Geometry check sheet. Reference: the model listing, model coordinates, mm. A direction names the side the tool comes from. Round coordinates to 2 decimals unless told otherwise and drop trailing zeros. Order: outer loops, then holes, each group sorted by start corner. A loop starts at its lowest first (then second) coordinate and runs counter-clockwise, first axis right, second up. Notation, with made-up numbers: (32, 89) - (39, 89) arc R16 cw to (39, 119) - close; hole circle Ø4 at (45.25, 13.25). An arc over 180 degrees is marked (long way). Use a Markdown table: item, result. Add a question column.
(1) Section check A-A on y = 20. Give the number of separate pieces and of enclosed holes in the cut face, then the cut area to 3 significant figures.
(2) Gauge pin test, flat ends, axial feed: P1, Ø6, axis at y = 24.5, z = -17.5, coming from the +X side; P2, Ø1.5, axis at y = 22.5, z = -22, coming from the -X side; P3, Ø4, axis at y = 29, z = -3.5, coming from the +X side. Record the tip position at first contact, or that the pin passes through.
(3) Section check B-B on y = 3. Record the boundary of the cut face in (x, z), then the cut area to 3 significant figures.
(4) Mould release check, pull along Y, two halves, no side actions. Record for faces 6 (the face through (5.27, 8.1, -11.44)), 7 (the face through (58, 35, -13)), 8 (the face through (46, 3, -24.75)): released by +Y, released by -Y, zero draft, split by the parting line, or undercut.
(5) Thickness scan on line 1 along Z through (x, y) = (18.5, 3); line 2 along X through (y, z) = (9, -12.25); line 3 along X through (y, z) = (10.5, -19.75). Record the ranges inside material, lowest first. Write a range as [from, to].
(6) Access from +Z, -Z, +X, -X, +Y, -Y to the whole of each face (thin tool, end or side, straight path). Record for faces 1 (the face through (1.25, 2, -13)), 2 (the face through (53.27, 8.1, -11.44)), 3 (the face through (13.5, 13, -4)), 4 (the face through (54.5, 27.3, -15.3)), 5 (the face through (61.5, 13, -4)).
(7) Section check C-C on x = 9.5. Record the boundary of the cut face in (y, z).
```python
from build123d import *

# Parameters (mm, degrees)
SKETCH1_W            = 20
SKETCH1_H            = 26
SKETCH1_W_2          = 1.25
SKETCH1_H_2          = 15
BOSS_EXTRUDE5_DEPTH  = 5
SKETCH3_W            = 7
SKETCH3_H            = 26
BOSS_EXTRUDE6_DEPTH  = 40
CUT_EXTRUDE1_REACH   = 55.696
SKETCH5_R            = 11.2
SKETCH6_W            = 26
SKETCH6_H            = 5
BOSS_EXTRUDE8_DEPTH  = 14
SKETCH8_R            = 12
SKETCH8_R_2          = 7.5
BOSS_EXTRUDE9_DEPTH  = 2.5
SKETCH9_R            = 12
SKETCH9_R_2          = 7.5
BOSS_EXTRUDE10_DEPTH = 2.5
SKETCH7_W            = 12
SKETCH7_H            = 1.25
CUT_EXTRUDE2_DEPTH   = 10


with BuildPart() as part:
    # Sketch1 → Boss-Extrude5 (new body)
    with BuildSketch(Plane(origin=(0, 0, 0), x_dir=(1, 0, 0), z_dir=(0, 1, 0))):
        with Locations((10, 13)):
            Rectangle(SKETCH1_W, SKETCH1_H)
        with Locations((1.875, 13)):
            Rectangle(SKETCH1_W_2, SKETCH1_H_2, mode=Mode.SUBTRACT)
    boss_extrude5 = extrude(amount=BOSS_EXTRUDE5_DEPTH)

    # Sketch3 → Boss-Extrude6 (add)
    with BuildSketch(Plane(origin=(0, 5, 0), x_dir=(1, 0, 0), z_dir=(0, 1, 0))):
        with Locations((10, 13)):
            Rectangle(SKETCH3_W, SKETCH3_H)
    boss_extrude6 = extrude(amount=BOSS_EXTRUDE6_DEPTH)

    # Sketch5 → Cut-Extrude1 (cut, up to next)
    with BuildSketch(Plane(origin=(13.5, 0, 0), x_dir=(0, 0, -1), z_dir=(1, 0, 0)), mode=Mode.PRIVATE) as cut_extrude1_sk1:
        with Locations((13, 20)):
            Circle(SKETCH5_R)
    cut_extrude1_tool1 = extrude(cut_extrude1_sk1.sketch, amount=-CUT_EXTRUDE1_REACH, mode=Mode.PRIVATE) & part.part
    # Sketch5 → Cut-Extrude1 (cut, up to next)
    with BuildSketch(Plane(origin=(13.5, 0, 0), x_dir=(0, 0, -1), z_dir=(1, 0, 0)), mode=Mode.PRIVATE) as cut_extrude1_sk2:
        with BuildLine():
            Line((0, 27.483314774), (0, 45))
            Line((0, 45), (26, 45))
            Line((26, 45), (26, 27.483314774))
            ThreePointArc((26, 27.483314774), (13, 35), (0, 27.483314774))
        make_face()
    cut_extrude1_tool2 = extrude(cut_extrude1_sk2.sketch, amount=-CUT_EXTRUDE1_REACH, mode=Mode.PRIVATE) & part.part
    cut_extrude1_1 = cut_extrude1_tool1.solids().sort_by_distance((13.5, 20, -13))[0]
    add(cut_extrude1_1, mode=Mode.SUBTRACT)
    cut_extrude1_2 = cut_extrude1_tool2.solids().sort_by_distance((13.5, 38.725293, -13))[0]
    add(cut_extrude1_2, mode=Mode.SUBTRACT)
    cut_extrude1 = cut_extrude1_1 + cut_extrude1_2  # Cut-Extrude1 as one shape, for the pattern or mirror that repeats it

    # Sketch6 → Boss-Extrude8 (add)
    with BuildSketch(Plane(origin=(20, 0, 0), x_dir=(0, 0, -1), z_dir=(1, 0, 0))):
        with Locations((13, 2.5)):
            Rectangle(SKETCH6_W, SKETCH6_H)
    boss_extrude8 = extrude(amount=BOSS_EXTRUDE8_DEPTH)

    # Mirror5: Boss-Extrude5, Boss-Extrude6, Cut-Extrude1, Boss-Extrude8 across plane
    add(boss_extrude5.mirror(Plane.ZY.offset(-34)))
    add(boss_extrude6.mirror(Plane.ZY.offset(-34)))
    add(cut_extrude1.mirror(Plane.ZY.offset(-34)), mode=Mode.SUBTRACT)
    add(boss_extrude8.mirror(Plane.ZY.offset(-34)))

    # Sketch8 → Boss-Extrude9 (add)
    with BuildSketch(Plane.ZY.offset(-6.5)):
        with Locations(Location((-13, 20, 0), (0, 0, 180))):
            Circle(SKETCH8_R)
        with Locations((-13, 20)):
            Circle(SKETCH8_R_2, mode=Mode.SUBTRACT)
    extrude(amount=BOSS_EXTRUDE9_DEPTH)

    # Sketch9 → Boss-Extrude10 (add)
    with BuildSketch(Plane.ZY.offset(-54.5)):
        with Locations(Location((-13, 20, 0), (0, 0, 180))):
            Circle(SKETCH9_R)
        with Locations((-13, 20)):
            Circle(SKETCH9_R_2, mode=Mode.SUBTRACT)
    extrude(amount=BOSS_EXTRUDE10_DEPTH)

    # Sketch7 → Cut-Extrude2 (cut)
    with BuildSketch(Plane(origin=(0, 5, 0), x_dir=(1, 0, 0), z_dir=(0, 1, 0))):
        with Locations((22, 1.875)):
            Rectangle(SKETCH7_W, SKETCH7_H)
        with Locations((46, 1.875)):
            Rectangle(SKETCH7_W, SKETCH7_H)
        with Locations((46, 24.125)):
            Rectangle(SKETCH7_W, SKETCH7_H)
        with Locations((22, 24.125)):
            Rectangle(SKETCH7_W, SKETCH7_H)
    extrude(amount=-CUT_EXTRUDE2_DEPTH, mode=Mode.SUBTRACT)


solid = part.part
```
Check sheet entries:
| question | item | result |
|---|---|---|
| 1 | separate pieces | 4 |
| 1 | enclosed holes | 0 |
| 1 | area | 95.4 mm2 |
| 2 | P1 | stops at x = 54.5 |
| 2 | P2 | stops at x = 4 |
| 2 | P3 | stops at x = 61.5 |
| 3 | outline | (0, -26) - (68, -26) - (68, 0) - (0, 0) - close; hole (1.25, -20.5) - (2.5, -20.5) - (2.5, -5.5) - (1.25, -5.5) - close; hole (16, -24.75) - (28, -24.75) - (28, -23.5) - (16, -23.5) - close; hole (16, -2.5) - (28, -2.5) - (28, -1.25) - (16, -1.25) - close; hole (40, -24.75) - (52, -24.75) - (52, -23.5) - (40, -23.5) - close; hole (40, -2.5) - (52, -2.5) - (52, -1.25) - (40, -1.25) - close; hole (65.5, -20.5) - (66.75, -20.5) - (66.75, -5.5) - (65.5, -5.5) - close |
| 3 | area | 1,670 mm2 |
| 4 | face 6 | undercut |
| 4 | face 7 | released by +Y |
| 4 | face 8 | zero draft |
| 5 | line 1 | z = [-26, -24.75], [-23.5, -2.5], [-1.25, 0] |
| 5 | line 2 | x = [4, 6.5], [52, 54.5] |
| 5 | line 3 | x = [4, 13.5], [52, 61.5] |
| 6 | face 1 | +Y, -Y |
| 6 | face 2 | none |
| 6 | face 3 | +Z, -Z, +Y |
| 6 | face 4 | +X |
| 6 | face 5 | +Z, -Z, +X, +Y |
| 7 | outline | (0, -26) - (27.48, -26) arc R15 ccw to (27.48, 0) - (0, 0) - close; hole circle Ø22.4 at (20, -13) |
